Geometry: see drawing. Coordinates: mm, zero at the bounding-box minimum. A direction names the side the tool comes from. Coordinates: 2 decimals unless noted, no trailing zeros. Order: outer loops, then holes, each group sorted by start corner. A loop starts at its lowest first (then second) coordinate and runs counter-clockwise, first axis right, second up.
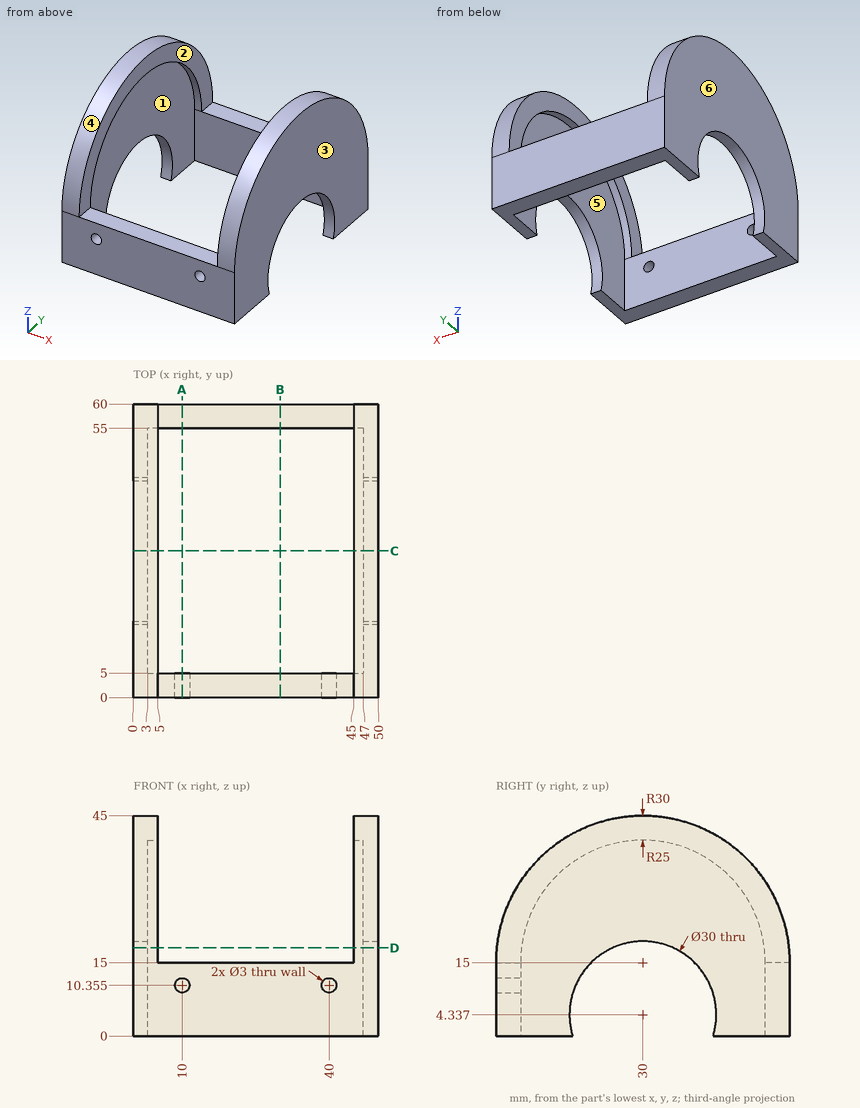
Item 1: Ray query, probe 1 along Y at (x, z) = (41, 6); probe 2 along X at (y, z) = (10, 25.5); probe 3 along X at (y, z) = (52, 35). Return the intervals inside material, ascending.
Response values:
probe 1: y = 0 to 5, 55 to 60
probe 2: x = 0 to 3, 47 to 50
probe 3: x = 0 to 5, 45 to 50
Item 2: Cut plane A-A on x = 10. Return loops of the section in (y, z) (3 decimals), then the cut area to 3 significant figures.
Response values:
outline: (0, 0) - (5, 0) - (5, 8.855) - (0, 8.855) - close; (0, 11.855) - (5, 11.855) - (5, 15) - (0, 15) - close; (55, 0) - (60, 0) - (60, 15) - (55, 15) - close
area: 135 mm2
Item 3: Cut plane B-B on x = 30. Return loops of the section in (y, z), then the cut area to 3 significant figures.
Response values:
outline: (0, 0) - (5, 0) - (5, 15) - (0, 15) - close; (55, 0) - (60, 0) - (60, 15) - (55, 15) - close
area: 150 mm2
Item 4: Pin query (flat end, axial travel): pin 1 Ø1.5 at (x, y) = (29.5, 1.5) entering from +Z; pin 2 Ø1.8 at (x, z) = (40, 10.355) entering from -Y. Return the tip coordinate at first contact, or that it passes through.
Response values:
pin 1: stops at z = 15
pin 2: stops at y = 55
Item 5: Cut plane C-C on y = 30. Return loops of the section in (x, z), then the cut area to 3 significant figures.
Response values:
outline: (0, 19.34) - (3, 19.34) - (3, 40) - (5, 40) - (5, 45) - (0, 45) - close; (45, 40) - (47, 40) - (47, 19.34) - (50, 19.34) - (50, 45) - (45, 45) - close
area: 174 mm2
Item 6: Draft query along Y for the marked faces 4, 5 and 6. Return one class per face: pulls with the +Y half, pulls with the -Y half, needs draft (parallel to the pull), parting line crosses it, or undercut.
Response values:
face 4: parting line crosses it
face 5: undercut
face 6: needs draft
Item 7: Cut plane D-D on z = 18. Return loops of the section in (x, y).
Response values:
outline: (0, 0.15) - (5, 0.15) - (5, 5.18) - (3, 5.18) - (3, 23.81) - (0, 23.81) - close; (0, 36.19) - (3, 36.19) - (3, 54.82) - (5, 54.82) - (5, 59.85) - (0, 59.85) - close; (45, 0.15) - (50, 0.15) - (50, 23.81) - (47, 23.81) - (47, 5.18) - (45, 5.18) - close; (45, 54.82) - (47, 54.82) - (47, 36.19) - (50, 36.19) - (50, 59.85) - (45, 59.85) - close
Item 8: Access query for the marked faces 1, 2 and 3. Directions: +Z, -Z, +X, -X, +Y, -Y. A direction counts if a zero-diameter tool reaches every point of the face in a straight line with its end or side. Return the directions, or none.
Response values:
face 1: -Z
face 2: +Z, +Y, -Y
face 3: +Z, -Z, +X, +Y, -Y
